Source: CAD feature listing. Evaluate the final solid. Frame: model axes, mm. Face numbers are marked on the shaded views. A direction names the side the tool comes from. Coordinates: 2 decimals unless noted, no trailing zeros. Order: outer loops, then holes, each group sorted by start corner. A loop starts at its lowest first (then second) coordinate and runs counter-clockwise, first axis right, second up.
Item 1: Section C-C on z = -2.5. Return the cut outline in (x, y) (3 decimals), then the cut area to 3 significant figures.
Item 2: Mould query, pull axis Z, two halves, no side actions, for the marked faces 6, 7, 8 and 9. Classes: released by +Z, released by -Z, zero draft, split by the parting line, or undercut.
Item 3: Section D-D on x = -12. Return the cut outline in (y, z) (3 decimals), then the cut area to 3 significant figures.
Item 4: Contact query for flat-ended pins moving along their axis: P1, Ø4, axis at y = 8.5, z = 4.5, coming from the -X side (3 decimals); P2, Ø3, axis at x = -12.5, z = -2.5, coming from the +Y side (3 decimals); P3, Ø5, axis at x = -8.62, z = -6.35, coming from the -Y side; P4, Ø0.6, axis at x = -3, z = -2, coming from the +Y side (3 decimals). Output: stop coordinate, or through.
Item 5: Reachability of the marked faces 1, 2, 3, 4 and 5 from +Z, -Z, +X, -X, +Y, -Y: full face, straight path, thin tool, end or side. Return the list, or none.
Item 6: Section B-B on y = 12.25. Return the cut outline in (x, z) (3 decimals).
Item 7: Ray query, line 1 (Z direction, x = -8.62, y = 0.65) (3 decimals); line 2 (Z direction, x = -1, y = 9) (3 decimals); line 3 (X direction, y = 1.5, z = -6.35) (3 decimals). Return the intervals inside material, ascending.
Item 8: Section A-A on y = 6.35. Return the cut outline in (x, z) (3 decimals).
from build123d import *

# Parameters (mm, degrees)
BOSS_EXTRUDE1_DEPTH = 10.795
SKETCH2_R           = 0.889
SKETCH2_W           = 10.16
SKETCH2_H           = 12.7
CUT_EXTRUDE1_DEPTH  = 16.875
SKETCH3_R           = 1.6
CUT_EXTRUDE2_DEPTH  = 4.175
SKETCH5_W           = 1.175
SKETCH5_H           = 10.16
BOSS_EXTRUDE2_DEPTH = 4
CHAMFER1_SIZE       = 0.254
FILLET1_R           = 2.54
FILLET2_R           = 1.27


with BuildPart() as part:
    # Sketch1 → Boss-Extrude1 (new body, symmetric)
    with BuildSketch(Plane.XY):
        Polygon((-15.875, 0), (0, 0), (0, 15.875), (-3.175, 15.875), (-3.175, 3.175), (-15.875, 3.175), align=None)
    extrude(amount=BOSS_EXTRUDE1_DEPTH, both=True)

    # Sketch2 → Cut-Extrude1 (cut, through all)
    with BuildSketch(Plane(origin=(0, 0, 0), x_dir=(0, 0, -1), z_dir=(1, 0, 0))):
        with Locations((-8.255, 6.35)):
            Circle(SKETCH2_R)
        with Locations((8.255, 6.35)):
            Circle(SKETCH2_R)
        with Locations((0, 9.525)):
            Rectangle(SKETCH2_W, SKETCH2_H)
    extrude(amount=-CUT_EXTRUDE1_DEPTH, mode=Mode.SUBTRACT)

    # Sketch3 → Cut-Extrude2 (cut, through all)
    with BuildSketch(Plane(origin=(0, 3.175, 0), x_dir=(1, 0, 0), z_dir=(0, 1, 0))):
        with Locations((-8.62, 6.35)):
            Circle(SKETCH3_R)
        with Locations((-8.62, -6.35)):
            Circle(SKETCH3_R)
    extrude(amount=-CUT_EXTRUDE2_DEPTH, mode=Mode.SUBTRACT)

    # Sketch5 → Boss-Extrude2 (add)
    with BuildSketch(Plane(origin=(0, 3.175, 0), x_dir=(1, 0, 0), z_dir=(0, 1, 0))):
        with Locations((-2.5875, 0)):
            Rectangle(SKETCH5_W, SKETCH5_H)
    extrude(amount=BOSS_EXTRUDE2_DEPTH)

    # Chamfer1
    chamfer1_edges = [part.edges().sort_by_distance(p)[0] for p in [
        (-10.22, 3.175, -6.35),
        (-10.22, 3.175, 6.35),
    ]]
    chamfer(chamfer1_edges, length=CHAMFER1_SIZE)

    # Fillet1
    fillet1_edges = [part.edges().sort_by_distance(p)[0] for p in [
        (-1.5875, 15.875, 10.795),
        (-15.875, 1.5875, 10.795),
        (-1.5875, 15.875, -10.795),
        (-15.875, 1.5875, -10.795),
    ]]
    fillet(fillet1_edges, radius=FILLET1_R)

    # Fillet2
    fillet2_edges = [part.edges().sort_by_distance(p)[0] for p in [
        (-1.5875, 15.875, 5.08),
        (-1.5875, 15.875, -5.08),
    ]]
    fillet(fillet2_edges, radius=FILLET2_R)


solid = part.part
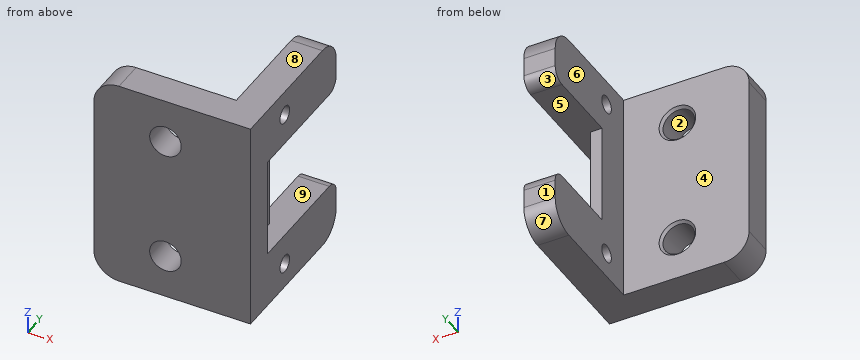
Answer list:
1. outline: (-15.875, 0) - (0, 0) - (0, 3.175) - (-2, 3.175) - (-2, 7.175) - (-3.175, 7.175) - (-3.175, 3.175) - (-15.875, 3.175) - close
1. area: 55.1 mm2
2. face 6: zero draft
2. face 7: released by -Z
2. face 8: released by +Z
2. face 9: undercut
3. outline: (0, -10.795) - (3.175, -10.795) - (3.175, 10.795) - (0, 10.795) - close
3. area: 68.5 mm2
4. P1: stops at x = -3.175
4. P2: stops at y = 3.175
4. P3: stops at y = 0
4. P4: stops at y = 7.175
5. face 1: +Z, -Z, +X, -X, +Y
5. face 2: +Y, -Y
5. face 3: +X, -X, +Y
5. face 4: +Z, -Z, -X, +Y
5. face 5: +X, +Y
6. outline: (-3.175, -10.795) - (0, -10.795) - (0, -5.08) - (-3.175, -5.08) - close; (-3.175, 5.08) - (0, 5.08) - (0, 10.795) - (-3.175, 10.795) - close
7. line 1: z = -10.795 to -7.95, -4.75 to 4.75, 7.95 to 10.795
7. line 2: z = -10.795 to -5.08, 5.08 to 10.795
7. line 3: x = -15.875 to -10.22, -7.02 to 0
8. outline: (-3.175, -10.795) - (0, -10.795) - (0, -9.144) - (-3.175, -9.144) - close; (-3.175, -7.366) - (0, -7.366) - (0, -5.08) - (-2, -5.08) - (-2, 5.08) - (0, 5.08) - (0, 7.366) - (-3.175, 7.366) - close; (-3.175, 9.144) - (0, 9.144) - (0, 10.795) - (-3.175, 10.795) - close
